The listing builds one solid part. Answer for the finished solid, in the listing's coordinates (mm). A direction names the side the tool comes from. Give positions to 0.01 mm unless a question says otherwise; leave off trailing zeros. Order: outer loops, then holes, each group sorted by start corner. A loop starts at its lowest first (then second) coordinate and runs counter-clockwise, first axis right, second up. Notation, with made-up numbers: (38.25, -11.5) - (94.25, -11.5) arc R21 cw to (94.25, 23.5) - close; hole circle Ø5 at (13, 83.25). An arc over 180 degrees is marked (long way). Use a Markdown table: item, result. Add a question column.
1) Find section B-B, the plane y = 0.75. Determine the outline of the cut face in (x, z).
2) The mould has two halves that part along Z. Classify faces 6 (the face through (-18.45, 4, -45)), 7 (the face through (0, 3, -45)), 8 (the face through (-20, 3, -60)): released by +Z, released by -Z, zero draft, split by the parting line, or undercut.
3) Straight lines are drawn through the part: line 1 (Z direction, x = -20, y = 5.95); line 2 (X direction, y = 5.55, z = -45); line 3 (X direction, y = 3.5, z = -35.25). For each, find the intervals that lie inside material, in ascending order.
4) Flat-ended cylindrical pins translate along their axes: pin 1 (4 mm diameter, centred on x = -10, z = -27.5, fed in from +Y); pin 2 (3.5 mm diameter, centred on x = -19.5, y = 3.5, fed in from +Z); pin 3 (0.9 mm diameter, centred on x = -20, z = -45.5, fed in from +Y); pin 4 (3.5 mm diameter, centred on y = 5, z = -16.5, fed in from +X). Find the tip coordinate at first contact, or state that the pin passes through.
5) Find section C-C, the plane z = -22. Determine the outline of the cut face in (x, y), plus the area to 3 significant figures.
6) For faces 1 (the face through (-21.38, 3.95, -36.82)), 2 (the face through (-13, 4, -30)), 3 (the face through (-24, 7, -36)), 4 (the face through (-24, 0, -36)), 5 (the face through (-21.55, 4, -45)), determine the directions among +Z, -Z, +X, -X, +Y, -Y from which every point of the face is accessible in a straight line to the end or side of a thin tool.
7) Find section A-A, the plane z = -45. Determine the outline of the cut face in (x, y), plus the area to 3 significant figures.
Autodesk Inventor part; units mm, degrees
ref_plane "YZ Plane" through (0, 0, 0) normal (1, 0, 0) x (0, 1, 0)
ref_plane "XZ Plane" through (0, 0, 0) normal (0, 1, 0) x (-1, 0, 0)
ref_plane "XY Plane" through (0, 0, 0) normal (0, 0, 1) x (1, 0, 0)
sketch "Sketch1" plane through (0, 0, 0) normal (0, 1, 0) x (-1, 0, 0)
  line L0 (0, 0) -> (40, 0)
  line L1 (40, 0) -> (40, -60)
  line L2 (40, -60) -> (0, -60)
  line L3 (0, -60) -> (0, 0)
  dimension "d0" = 40
  dimension "d1" = 60
extrude "Extrusion1" add sketch "Sketch1" along normal blind 7
sketch "Sketch2" plane through (0, 7, 0) normal (0, 1, 0) x (1, 0, 0)
  line L0 (-40, 0) -> (0, 0)
  line L1 (0, 0) -> (-25.544, 0)
  line L2 (-25.544, 0) -> (-25.544, 30)
  line L3 (-25.544, 30) -> (0, 30)
  line L4 (0, 30) -> (0, 0)
  dimension "d4" = 25.544
  dimension "d5" = 30
extrude "Extrusion2" cut sketch "Sketch2" against normal through all
sketch "Sketch3" plane through (0, 7, 0) normal (0, 1, 0) x (1, 0, 0)
  circle A0 centre (-20, 45) radius 6.4
  point P0 (0, 0)
  dimension "d8" = 12.8
extrude "Extrusion3" cut sketch "Sketch3" against normal blind 2
sketch "Sketch4" plane through (-20, 5, -45) normal (0, 1, 0) x (1, 0, 0)
  line L0 (-1.55, -1.55) -> (1.55, -1.55)
  line L1 (1.55, -1.55) -> (1.55, 1.55)
  line L2 (1.55, 1.55) -> (-1.55, 1.55)
  line L3 (-1.55, 1.55) -> (-1.55, -1.55)
  line L4 (-1.55, -1.55) -> (1.55, 1.55) construction
  line L5 (1.55, -1.55) -> (-1.55, 1.55) construction
  point P0 (20, -45)
  point P1 (0, 0)
  dimension "d11" = 3.1
  dimension "d12" = 3.1
extrude "Extrusion4" cut sketch "Sketch4" against normal blind 3
sketch "Sketch6" plane through (-18.45, 5, -43.45) normal (0, 0, -1) x (-1, 0, 0)
  circle A0 centre (1.5, -1.5) radius 1.5
  point P0 (-18.45, -5)
  dimension "d18" = 3
extrude "Extrusion6" cut sketch "Sketch6" against normal through all
The answers:
| question | item | result |
|---|---|---|
| 1 | outline | (-40, -60) - (0, -60) - (0, -30) - (-25.54, -30) - (-25.54, 0) - (-40, 0) - close |
| 2 | face 6 | undercut |
| 2 | face 7 | zero draft |
| 2 | face 8 | released by -Z |
| 3 | line 1 | -60 to -51.4, -38.6 to -30 |
| 3 | line 2 | -40 to -26.4, -13.6 to 0 |
| 3 | line 3 | -40 to -21.45, -18.45 to 0 |
| 4 | pin 1 | through |
| 4 | pin 2 | z = -30 |
| 4 | pin 3 | y = 2 |
| 4 | pin 4 | x = -25.54 |
| 5 | outline | (-40, 0) - (-25.54, 0) - (-25.54, 7) - (-40, 7) - close |
| 5 | area | 101 mm2 |
| 6 | face 1 | +Z |
| 6 | face 2 | +Z, +X, +Y, -Y |
| 6 | face 3 | +Z, -Z, +X, -X, +Y |
| 6 | face 4 | +Z, -Z, +X, -X, -Y |
| 6 | face 5 | +Y |
| 7 | outline | (-40, 0) - (0, 0) - (0, 7) - (-13.6, 7) - (-13.6, 5) - (-18.45, 5) - (-18.45, 2) - (-21.55, 2) - (-21.55, 5) - (-26.4, 5) - (-26.4, 7) - (-40, 7) - close |
| 7 | area | 245 mm2 |
